Could you check a few things on this model? Use its own coordinates, in mm. A direction names the side the tool comes from. Give positions to 0.01 mm unless a question says otherwise; leave off trailing zeros. Order: outer loops, then holes, each group sorted by start corner. A loop starts at its lowest first (then second) coordinate and runs counter-clockwise, first axis right, second up.
Autodesk Inventor part; units mm, degrees
ref_plane "YZ Plane" through (0, 0, 0) normal (1, 0, 0) x (0, 1, 0)
ref_plane "XZ Plane" through (0, 0, 0) normal (0, 1, 0) x (-1, 0, 0)
ref_plane "XY Plane" through (0, 0, 0) normal (0, 0, 1) x (1, 0, 0)
sketch "Sketch1" plane through (0, 0, 0) normal (0, 0, 1) x (1, 0, 0)
  circle A0 centre (0, 0) radius 48.5902 construction
  circle A1 centre (0, 0) radius 42.1132 construction
  circle A2 centre (0, 0) radius 54.61
  circle A3 centre (0, 0) radius 51.7652 construction
  line L0 (0, 0) -> (0, 45.3517) construction
  line L1 (-25.4, -25.4) -> (25.4, -25.4)
  line L2 (25.4, -25.4) -> (25.4, 25.4)
  line L3 (25.4, 25.4) -> (-25.4, 25.4)
  line L4 (-25.4, 25.4) -> (-25.4, -25.4)
  line L5 (-25.4, -25.4) -> (25.4, 25.4) construction
  line L6 (25.4, -25.4) -> (-25.4, 25.4) construction
  dimension "d0" = 97.1804
  dimension "d1" = 84.2264
  dimension "d2" = 109.22
  dimension "d3" = 103.5304
  dimension "d15" = 45.3517
  dimension "d22" = 50.8
  dimension "d23" = 50.8
sketch "Sketch2" plane through (0, 0, 0) normal (1, 0, 0) x (0, 1, 0)
  line L0 (0, 0) -> (45.3517, 0) construction
  line L1 (45.3517, 0) -> (45.3517, 0.7937) construction
  circle A0 centre (45.3517, 0.7937) radius 3.2385
  line L2 (0, 0) -> (0, 25.4) construction
  dimension "d16" = 6.477
  dimension "d17" = 0.7937
  dimension "d18" = 25.4
extrude "Extrusion2" add sketch "Sketch1" against normal blind 9.525
revolve "Revolution2" cut sketch "Sketch2" angle 360 about axis through (0, 0, 0) along (0, 0, 1)
equation "\"d15\" = 0.25 * d1 + 0.25 * d0"
properties part number "Base Gear" material "Aluminum 6061"
Item 1: For pin 1 (1 mm diameter, centred on x = 27.5, z = -3.5, fed in from +Y); pin 2 (4 mm diameter, centred on x = 17.5, z = -4, fed in from -Y); pin 3 (3 mm diameter, centred on x = 39.5, y = 36, fed in from +Z); pin 4 (1.5 mm diameter, centred on x = 16.5, z = -7, fed in from +Y), each with a flat end and sliding along its axis, tell me the tip position at first contact or that it passes through.
Findings:
pin 1: stops at y = 47.47
pin 2: stops at y = -52.36
pin 3: stops at z = 0
pin 4: stops at y = 52.29
Item 2: Imagine slicing it at A-A on x = 0. List the corners of the cut face in (y, z) for me (1 decimal).
Findings:
outline: (-54.6, -9.5) - (-25.4, -9.5) - (-25.4, 0) - (-42.2, 0) arc R3.2 cw to (-48.5, 0) - (-54.6, 0) - close; (25.4, -9.5) - (54.6, -9.5) - (54.6, 0) - (48.5, 0) arc R3.2 cw to (42.2, 0) - (25.4, 0) - close
Item 3: Imagine slicing it at C-C on z = -5. List the corners of the cut face in (x, y) for me.
Findings:
outline: circle Ø109.22 at (0, 0); hole (-25.4, -25.4) - (25.4, -25.4) - (25.4, 25.4) - (-25.4, 25.4) - close
Item 4: We'd pull the mould along Y, two halves only. Please class faces 1 (the cylindrical face through (-7.109, 54.145, -4.696)), 2 (the flat face through (-25.4, 0, -5)), 3 (the flat face through (36, 1, -9.525)): +Y half, -Y half, draft (parallel to the pull), parting line (faces both ways), or undercut.
Findings:
face 1: parting line
face 2: undercut
face 3: draft
Item 5: Please list where these lines run through material, in increasing order: line 1 along Y through (x, z) = (-31, -1); line 2 along X through (y, z) = (0.5, -3.75); line 3 along X through (y, z) = (-28.5, -0.25).
Findings:
line 1: y = -44.96 to -36.71, -29.3 to 29.3, 36.71 to 44.96
line 2: x = -54.61 to -25.4, 25.4 to 54.61
line 3: x = -46.58 to -39.14, -31.24 to 31.24, 39.14 to 46.58
Item 6: For faces 4 (the flat face through (0, 49, 0)), 5 (the flat face through (0, 25.4, -5)), which set-ups out of +Z, -Z, +X, -X, +Y, -Y let a thin tool reach every point of the face, with its end or its side?
Findings:
face 4: +Z, +X, -X, +Y, -Y
face 5: +Z, -Z
